```python
from build123d import *

# Parameters (mm, degrees)
F0_R     = 6.35
F1_DEPTH = 6.35
F2_R     = 3.175
F3_R     = 5.08
F4_R     = 3.175
F5_R     = 3.175


# Not quite as in the source:
# - ends of sketch curves that miss each other by under 0.0002 mm in the source are joined


with BuildPart() as f1:
    # F0 (on Front) → F1 (new body)
    with BuildSketch(Plane.XZ):
        with BuildLine():
            Line((-72.7094654823, -50.272475262), (-83.3648741359, -50.272475262))
            ThreePointArc((-83.3648741359, -50.272475262), (-100.4842470659, -51.222143603), (-101.056400417, -68.3582903151))
            Line((-101.056400417, -68.3582903151), (-80.147210941, -92.8018072064))
            Line((-80.147210941, -92.8018072064), (-80.147210941, -134.409975262))
            Line((-80.147210941, -134.409975262), (262.752789059, -134.409975262))
            Line((262.752789059, -134.409975262), (262.752789059, -96.309975262))
            Line((262.752789059, -96.309975262), (256.402789059, -96.309975262))
            Line((256.402789059, -96.309975262), (256.402789059, -102.659975262))
            Line((256.402789059, -102.659975262), (250.052789059, -102.659975262))
            Line((250.052789059, -102.659975262), (250.052789059, -96.309975262))
            Line((250.052789059, -96.309975262), (231.002789059, -96.309975262))
            Line((231.002789059, -96.309975262), (231.002789059, -102.659975262))
            Line((231.002789059, -102.659975262), (224.652789059, -102.659975262))
            Line((224.652789059, -102.659975262), (224.652789059, 43.390024738))
            Line((224.652789059, 43.390024738), (218.302789059, 43.390024738))
            Line((218.302789059, 43.390024738), (218.302789059, 62.440024738))
            Line((218.302789059, 62.440024738), (224.652789059, 62.440024738))
            Line((224.652789059, 62.440024738), (224.652789059, 81.490024738))
            Line((224.652789059, 81.490024738), (61.4126609984, 81.490024738))
            Line((61.4126609984, 81.490024738), (56.0792184251, 76.1565821646))
            Line((56.0792184251, 76.1565821646), (60.5693464856, 71.6664541041))
            Line((60.5693464856, 71.6664541041), (6.8929171195, 17.990024738))
            Line((6.8929171195, 17.990024738), (123.052789059, 17.990024738))
            ThreePointArc((123.052789059, 17.990024738), (158.9738135432, 3.1110492223), (173.852789059, -32.809975262))
            Line((173.852789059, -32.809975262), (173.852789059, -45.509975262))
            ThreePointArc((173.852789059, -45.509975262), (158.9738135432, -81.4309997463), (123.052789059, -96.309975262))
            Line((123.052789059, -96.309975262), (81.777789059, -96.309975262))
            Line((81.777789059, -96.309975262), (81.777789059, -102.659975262))
            Line((81.777789059, -102.659975262), (62.727789059, -102.659975262))
            Line((62.727789059, -102.659975262), (62.727789059, -96.309975262))
            Line((62.727789059, -96.309975262), (-3.947210941, -96.309975262))
            Line((-3.947210941, -96.309975262), (-3.947210941, -102.659975262))
            Line((-3.947210941, -102.659975262), (-10.297210941, -102.659975262))
            Line((-10.297210941, -102.659975262), (-10.297210941, -96.309975262))
            Line((-10.297210941, -96.309975262), (-29.347210941, -96.309975262))
            Line((-29.347210941, -96.309975262), (-29.347210941, -102.659975262))
            Line((-29.347210941, -102.659975262), (-35.697210941, -102.659975262))
            Line((-35.697210941, -102.659975262), (-35.697210941, -96.309975262))
            Line((-35.697210941, -96.309975262), (-42.047210941, -96.309975262))
            Line((-42.047210941, -96.309975262), (-42.047210941, -50.272475262))
            Line((-42.047210941, -50.272475262), (-49.4849563998, -50.272475262))
            Line((-49.4849563998, -50.272475262), (-61.097210941, -60.0163137647))
            Line((-61.097210941, -60.0163137647), (-72.7094654823, -50.272475262))
        make_face()
        with Locations((-91.4055753496, -60.1028935639)):
            Circle(F0_R, mode=Mode.SUBTRACT)
    extrude(amount=-F1_DEPTH)

    # F2
    f2_edges = [f1.edges().sort_by_distance(p)[0] for p in [
        (224.652789, 3.175, 81.490025),
        (-42.047211, 3.175, -96.309975),
    ]]
    fillet(f2_edges, radius=F2_R)

    # F3
    f3_edges = [f1.edges().sort_by_distance(p)[0] for p in [
        (-80.147211, 3.175, -92.801807),
    ]]
    fillet(f3_edges, radius=F3_R)

    # F4
    f4_edges = [f1.edges().sort_by_distance(p)[0] for p in [
        (-42.047211, 3.175, -50.272475),
    ]]
    fillet(f4_edges, radius=F4_R)

    # F5
    f5_edges = [f1.edges().sort_by_distance(p)[0] for p in [
        (-61.097211, 3.175, -60.016314),
        (-83.364874, 3.175, -50.272475),
        (262.752789, 3.175, -96.309975),
    ]]
    fillet(f5_edges, radius=F5_R)


solid = f1.part
```
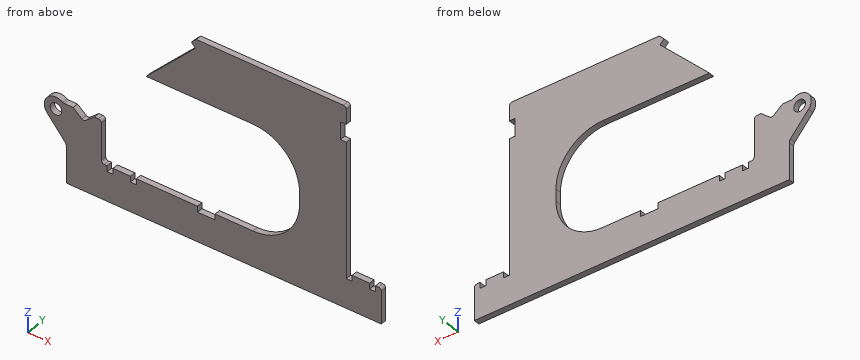
Read the model definition and answer for the solid it produces. Units are mm, in the model's axes. Give positions to 0.01 mm unless a question says otherwise; leave off trailing zeros. Write each loop counter-clockwise with the first axis right and the second up, starting at its lowest first coordinate (ties: lowest second). Pieces come first, ordered by that corner, then holes. Notation, with made-up numbers: (-0.5, 80.25) - (28.5, 80.25) arc R8 cw to (28.5, 84.25) - close; hole circle Ø7 at (73, 77). An arc over 180 degrees is marked (long way). Write item = value, one per line. Start each with the question number.
Item 1: Each of these flat-tipped pins is pushed along its axis until it touches: P1, Ø1.9, axis at y = 2.5, z = -100.5, coming from the -X side; P2, Ø1.9, axis at y = 4.5, z = 69, coming from the +X side; P3, Ø1.9, axis at x = -79.5, y = 4.5, coming from the +Z side. Where does it stop, or does it pass through?
Item 2: Find section B-B (z = -74.5). Give the vertices of the cut face in (x, y), then the cut area to 3 significant figures.
Item 3: Find section C-C (x = -17). Give the vertices of the cut face in (y, z), then the cut area to 3 significant figures.
Item 4: Find the intervals of material crossed by probe 1 along Z at (x, y) = (64, 2.5); probe 2 along Z at (x, y) = (82, 1.75); probe 3 along X at (y, z) = (4.75, -63), in increasing order. Write a range as [from, to].
Item 5: Find section A-A (x = 72). Give the vertices of the cut face in (y, z), then the cut area to 3 significant figures.
Item 6: Find section D-D (z = -39.5). Give the vertices of the cut face in (x, y).
Response:
q1.P1 = -80.15
q1.P2 = 224.65
q1.P3 = -50.27
q2.outline = (-95.8, 0) - (-42.05, 0) - (-42.05, 6.35) - (-95.8, 6.35) - close; (164.77, 0) - (224.65, 0) - (224.65, 6.35) - (164.77, 6.35) - close
q2.area = 722 mm²
q3.outline = (0, -134.41) - (6.35, -134.41) - (6.35, -96.31) - (0, -96.31) - close
q3.area = 242 mm²
q4.probe_1 = [-134.41, -102.66], [17.99, 81.49]
q4.probe_2 = [-134.41, -96.31], [17.99, 81.49]
q4.probe_3 = [-103.77, -97.06], [-85.75, -42.05], [170.75, 224.65]
q5.outline = (0, -134.41) - (6.35, -134.41) - (6.35, -102.66) - (0, -102.66) - close; (0, 17.99) - (6.35, 17.99) - (6.35, 81.49) - (0, 81.49) - close
q5.area = 605 mm²
q6.outline = (173.85, 0) - (224.65, 0) - (224.65, 6.35) - (173.85, 6.35) - close
